from build123d import *

# Parameters (mm, degrees)
F0_R     = 1.27
F1_DEPTH = 30.48
F3_DEPTH = 2.54
F5_D     = 1.27
F6_R     = 0.5728725826
F7_DEPTH = 0.3302


# Not quite as in the source:
# - a feature names something its author has since deleted; it is built from what else it names


with BuildPart() as f1:
    # F0 (on Front) → F1 (new body)
    with BuildSketch(Plane.XZ):
        with Locations((-44.9135862291, 42.5175279379)):
            Circle(F0_R)
    extrude(amount=F1_DEPTH)

    # F2 (on face) → F3 (join)
    with BuildSketch(Plane(origin=(0, 0, 0), x_dir=(-1, 0, 0), z_dir=(0, 1, 0))):
        Polygon((44.2763268948, 43.6160726756), (44.2763268948, 42.5175279379), (44.2763268948, 41.4189832001), (45.5469042063, 41.4189832001), (45.5469042063, 43.6183496036), align=None)
    extrude(amount=F3_DEPTH)

    # F5 (through all)
    with Locations(Plane(origin=(-45.5469042063, 0, 0), x_dir=(0, -1, 0), z_dir=(-1, 0, 0))):
        with Locations((-1.5291915042, 42.6044538617)):
            Hole(F5_D / 2)

    # F6 (on face) → F7 (cut)
    with BuildSketch(Plane(origin=(0, 2.54, 0), x_dir=(-1, 0, 0), z_dir=(0, 1, 0))):
        with Locations((44.9116155505, 42.5175279379)):
            Circle(F6_R)
    extrude(amount=-F7_DEPTH, mode=Mode.SUBTRACT)


solid = f1.part
The model under review builds one solid part; all positions refer to its coordinate system, in mm. A direction names the side the tool comes from. Round coordinates to 2 decimals unless told otherwise and drop trailing zeros. Order: outer loops, then holes, each group sorted by start corner. A loop starts at its lowest first (then second) coordinate and runs counter-clockwise, first axis right, second up. Notation, with made-up numbers: (-39.5, 50) -> (1.5, 50) arc R20 ccw to (1.5, 66) -> close; hole circle Ø8 at (62.5, -38.5). An arc over 180 degrees is marked (long way). Use CSV: the item, a comma, the result in double quotes. Start each with the question number.
(1) Consider section A-A on x = -44.9. Write out the cut boundary in (y, z) (3 decimals).
(2) Wall thickness on probe 1 along Y at (x, z) = (-44.15, 43.3); probe 2 along X at (y, z) = (-10.5, 42.45); probe 3 along Y at (x, z) = (-45.2, 43.15): over which ranges is each line inside the solid? List them lowest first. Write a range as from..to.
(3) Mouldability with a two-part tool opening along X and no side actions: class faces 4 (the face through (-45.547, 1, 42)), 5 (the face through (-44.457, 2.377, 42.169)), 6 (the face through (-44.903, 1.392, 41.985)) as pulls with the +X half, pulls with the -X half, needs draft (parallel to the pull), parting line crosses it, or undercut.
(4) Insertion check: pin 1 (0.9 mm diameter, centred on x = -44.91, z = 42.52, fed in from +Y); pin 2 (0.7 mm diameter, centred on y = 1, z = 42.5, fed in from +X). Each pin has a flat end and moves straight along its axis. Give the tip position at first contact, or say it passes through.
(5) Consider section B-B on y = -5.5. Write out the cut boundary in (x, z), and give its area (3 significant figures).
(6) Tool access review of faces 1 (the face through (-44.276, 1, 42)), 2 (the face through (-45.7, 0, 42.4)), 3 (the face through (-45, 1, 41.419)): name each direction out of +Z, -Z, +X, -X, +Y, -Y from which nothing blocks a thin tool from reaching the whole face with its end or side.
Responses:
1,outline,"(-30.48, 41.248) -> (0, 41.248) -> (0, 41.419) -> (2.54, 41.419) -> (2.54, 41.945) -> (2.21, 41.945) -> (2.21, 43.09) -> (2.54, 43.09) -> (2.54, 43.617) -> (0, 43.617) -> (0, 43.787) -> (-30.48, 43.787) -> close; hole circle Ø1.27 at (1.529, 42.604)"
2,probe 1,"-30.48..0"
2,probe 2,"-46.18..-43.65"
2,probe 3,"-30.48..1.2, 1.85..2.54"
3,face 4,"pulls with the -X half"
3,face 5,"undercut"
3,face 6,"needs draft"
4,pin 1,"y = 2.21"
4,pin 2,"x = -44.28"
5,outline,"circle Ø2.54 at (-44.91, 42.52)"
5,area,"5.07 mm²"
6,face 1,"+Z, -Z, +X, +Y"
6,face 2,"-Z, -X, +Y"
6,face 3,"-Z, +X, -X, +Y"
